```python
from build123d import *

# Parameters (mm, degrees)
SKETCH1_W           = 36
SKETCH1_H           = 36
SKETCH1_R           = 1.6
BOSS_EXTRUDE1_DEPTH = 13
SKETCH2_W           = 15
SKETCH2_H           = 7.5
BOSS_EXTRUDE2_DEPTH = 8.5
SKETCH3_W           = 12
SKETCH3_H           = 1
BOSS_EXTRUDE3_DEPTH = 3


with BuildPart() as part:
    # Sketch1 → Boss-Extrude1 (new body)
    with BuildSketch(Plane(origin=(0, 0, 0), x_dir=(1, 0, 0), z_dir=(0, 1, 0))):
        Rectangle(SKETCH1_W, SKETCH1_H)
        with Locations(Location((-15.25, 15.25, 0), (0, 0, 90))):
            Circle(SKETCH1_R, mode=Mode.SUBTRACT)
        with Locations(Location((15.25, 15.25, 0), (0, 0, 90))):
            Circle(SKETCH1_R, mode=Mode.SUBTRACT)
        with Locations(Location((15.25, -15.25, 0), (0, 0, 90))):
            Circle(SKETCH1_R, mode=Mode.SUBTRACT)
        with Locations(Location((-15.25, -15.25, 0), (0, 0, 90))):
            Circle(SKETCH1_R, mode=Mode.SUBTRACT)
    extrude(amount=BOSS_EXTRUDE1_DEPTH)

    # Sketch2 → Boss-Extrude2 (add)
    with BuildSketch(Plane(origin=(18, 0, 0), x_dir=(0, 0, -1), z_dir=(1, 0, 0))):
        with Locations((4.5, 8.75)):
            Rectangle(SKETCH2_W, SKETCH2_H)
    extrude(amount=BOSS_EXTRUDE2_DEPTH)

    # Sketch3 → Boss-Extrude3 (add)
    with BuildSketch(Plane.XY.offset(18)):
        with Locations((4, 2.5)):
            Rectangle(SKETCH3_W, SKETCH3_H)
    extrude(amount=BOSS_EXTRUDE3_DEPTH)


solid = part.part
```
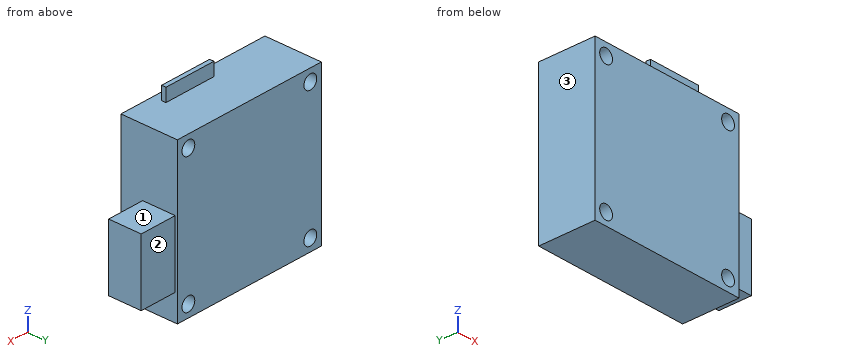
Input: part model. Units: mm. Frame: model coordinates. Face numbers are marked on the shaded views. A direction names the side the tool comes from. Give positions to 0.01 mm unless a question says otherwise; leave off trailing zeros. Loops run counter-clockwise (first coordinate to the right, second up) from the corner with the lowest first, then second, coordinate; pieces in that order, holes last. Notation, with made-up numbers: M 73.5,-21.75 L 125.5,-21.75 A7 cw 125.5,-15.75 Z; hole C 8,-5 d1. An arc over 180 degrees is marked long. Answer as CSV lines item,"result". Start each with the question number.
1. Section A-A on x = 15.25. Return loops of the section in (y, z).
2. Section D-D on z = -5. Return loops of the section in (x, y).
3. Reachability of the marked faces 1, 2 and 3 from +Z, -Z, +X, -X, +Y, -Y: full face, straight path, thin tool, end or side. Return the list, or none.
4. Pin query (flat end, axial travel): P1, Ø1.9, axis at x = -15.25, z = -15.25, coming from the +Y side; P2, Ø4, axis at y = 3.5, z = 8.5, coming from the +X side; P3, Ø0.9, axis at x = 3.5, z = 20, coming from the -Y side; P4, Ø0.5, axis at y = 2.5, z = 19.5, coming from the +X side. Return the tip coordinate at first contact, or that it passes through.
5. Section B-B on y = 7. Return loops of the section in (x, z).
6. Section C-C on z = -15.25. Return loops of the section in (x, y).
7. Line query: L1, parallel to Z at x = -15.25, y = 10.25; L2, parallel to Z at x = -6.5, y = 7.5. Output: solid intervals per line, ascending.
Computed values:
1,outline,"M 0,-18 L 13,-18 L 13,-16.85 L 0,-16.85 Z; M 0,-13.65 L 13,-13.65 L 13,13.65 L 0,13.65 Z; M 0,16.85 L 13,16.85 L 13,18 L 0,18 Z"
2,outline,"M -18,0 L 18,0 L 18,5 L 26.5,5 L 26.5,12.5 L 18,12.5 L 18,13 L -18,13 Z"
3,face 1,"+Z, +X, +Y, -Y"
3,face 2,"+Z, -Z, +X, +Y"
3,face 3,"+Z, -Z, -X, +Y, -Y"
4,P1,"passes through"
4,P2,"stops at x = 18"
4,P3,"stops at y = 2"
4,P4,"stops at x = 10"
5,outline,"M -18,-18 L 18,-18 L 18,-12 L 26.5,-12 L 26.5,3 L 18,3 L 18,18 L -18,18 Z; hole C -15.25,-15.25 d3.2; hole C -15.25,15.25 d3.2; hole C 15.25,-15.25 d3.2; hole C 15.25,15.25 d3.2"
6,outline,"M -18,0 L -16.85,0 L -16.85,13 L -18,13 Z; M -13.65,0 L 13.65,0 L 13.65,13 L -13.65,13 Z; M 16.85,0 L 18,0 L 18,13 L 16.85,13 Z"
7,L1,"z = -18 to -16.85, -13.65 to 13.65, 16.85 to 18"
7,L2,"z = -18 to 18"
